Here's how the part is built. I have some questions about the finished solid (model axes, mm). Face numbers are marked on the shaded views. A direction names the side the tool comes from. Give positions to 0.01 mm unless a question says otherwise; leave off trailing zeros. Write each loop counter-clockwise with the first axis right and the second up, starting at its lowest first coordinate (ties: lowest second). Pieces come first, ordered by that corner, then holes. Notation, with made-up numbers: (-10.75, 55.5) -> (2.25, 55.5) arc R29 cw to (2.25, 90.5) -> close; hole circle Ø10 at (63.25, -24.75). An arc over 180 degrees is marked (long way). Return JSON: item names as keys, results as strings.
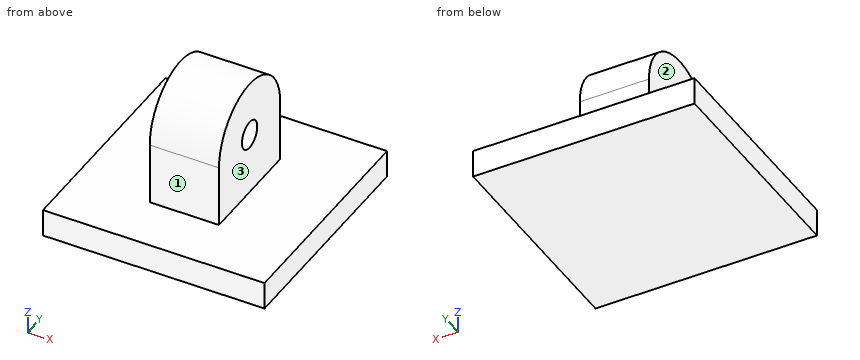
from build123d import *

# Parameters (mm, degrees)
SKETCH_1_W          = 16
SKETCH_1_H          = 16
EXTRUDE_1_DEPTH     = 2
SKETCH_2_W          = 5
SKETCH_2_H          = 8
EXTRUDE_2_DEPTH     = 4.5
SKETCH_3_R          = 4
EXTRUDE_3_DEPTH     = 5
SKETCH_4_R          = 1
CUT_EXTRUDE_1_DEPTH = 10


with BuildPart() as part:
    # 草图1 → 凸台-拉伸1 (new body)
    with BuildSketch(Plane.XY):
        with Locations((8, 8)):
            Rectangle(SKETCH_1_W, SKETCH_1_H)
    extrude(amount=EXTRUDE_1_DEPTH)

    # 草图2 → 凸台-拉伸2 (add)
    with BuildSketch(Plane.XY.offset(2)):
        with Locations((8, 8)):
            Rectangle(SKETCH_2_W, SKETCH_2_H)
    extrude(amount=EXTRUDE_2_DEPTH)

    # 草图3 → 凸台-拉伸3 (add)
    with BuildSketch(Plane.ZY.offset(-5.5)):
        with Locations((6.5, 8)):
            Circle(SKETCH_3_R)
    extrude(amount=-EXTRUDE_3_DEPTH)

    # 草图4 → 切除-拉伸1 (cut)
    with BuildSketch(Plane.ZY.offset(-5.5)):
        with Locations(Location((6.5, 8, 0), (0, 0, 270))):
            Circle(SKETCH_4_R)
    extrude(amount=-CUT_EXTRUDE_1_DEPTH, mode=Mode.SUBTRACT)


solid = part.part
1. For pin 1 Ø1.5 at (y, z) = (2, 4) entering from -X; pin 2 Ø4 at (y, z) = (13, 8.5) entering from +X; pin 3 Ø3 at (y, z) = (8, 6.5) entering from -X; pin 4 Ø1 at (x, z) = (7, 3) entering from +Y, each with a flat end and sliding along its axis, tell me the tip position at first contact or that it passes through.
Taken from the geometry:
{"pin 1": "passes through", "pin 2": "stops at x = 10.5", "pin 3": "stops at x = 5.5", "pin 4": "stops at y = 12"}
2. Suppose I cut it at A-A, the plane x = 9.75. List the corners of the cut face in (y, z) for me.
Taken from the geometry:
{"outline": "(0, 0) -> (16, 0) -> (16, 2) -> (12, 2) -> (12, 6.5) arc R4 ccw to (4, 6.5) -> (4, 2) -> (0, 2) -> close; hole circle Ø2 at (8, 6.5)"}
3. Suppose I cut it at C-C, the plane z = 6. List the corners of the cut face in (x, y) for me, and give its area (3 significant figures).
Taken from the geometry:
{"outline": "(5.5, 4) -> (10.5, 4) -> (10.5, 7.13) -> (5.5, 7.13) -> close; (5.5, 8.87) -> (10.5, 8.87) -> (10.5, 12) -> (5.5, 12) -> close", "area": "31.3 mm²"}
4. Suppose I cut it at B-B, the plane y = 8. List the corners of the cut face in (x, z) for me.
Taken from the geometry:
{"outline": "(0, 0) -> (16, 0) -> (16, 2) -> (10.5, 2) -> (10.5, 5.5) -> (5.5, 5.5) -> (5.5, 2) -> (0, 2) -> close; (5.5, 7.5) -> (10.5, 7.5) -> (10.5, 10.5) -> (5.5, 10.5) -> close"}
5. If I drill on line 1 (Z direction, x = 8.95, y = 8); line 2 (Z direction, x = 10.75, y = 14.25); line 3 (Y direction, x = 5.75, z = 6.25), over which ranges is the centre line in solid material (lowest first)? Write a range as [from, to].
Taken from the geometry:
{"line 1": "z = [0, 5.5], [7.5, 10.5]", "line 2": "z = [0, 2]", "line 3": "y = [4, 7.03], [8.97, 12]"}
6. Suppose I cut it at D-D, the plane y = 10. List the corners of the cut face in (x, z) for me, and give its area (3 significant figures).
Taken from the geometry:
{"outline": "(0, 0) -> (16, 0) -> (16, 2) -> (10.5, 2) -> (10.5, 9.96) -> (5.5, 9.96) -> (5.5, 2) -> (0, 2) -> close", "area": "71.8 mm²"}
7. Which directions (+Z, -Z, +X, -X, +Y, -Y) give clear straight access to the entire face, cutting with the end or side of a thin tool? Please do the marked faces 1, 2 and 3.
Taken from the geometry:
{"face 1": "+Z, +X, -X, -Y", "face 2": "+Z, -X, +Y, -Y", "face 3": "+Z, +X, +Y, -Y"}
